Geometry: see drawing. Coordinates: mm, zero at the bounding-box minimum. A direction names the side the tool comes from. Give positions to 0.01 mm unless a question says otherwise; leave off trailing zeros. Loops run counter-clockwise (first coordinate to the right, second up) from the corner with the lowest first, then second, coordinate; pieces in that order, holes last. Notation, with made-up numbers: M 80,-32 L 87,-32 A23 cw 87,-12 Z; hole C 57.5,-39 d7. An arc over 180 degrees is marked long. Answer in a Markdown table with one row per item.
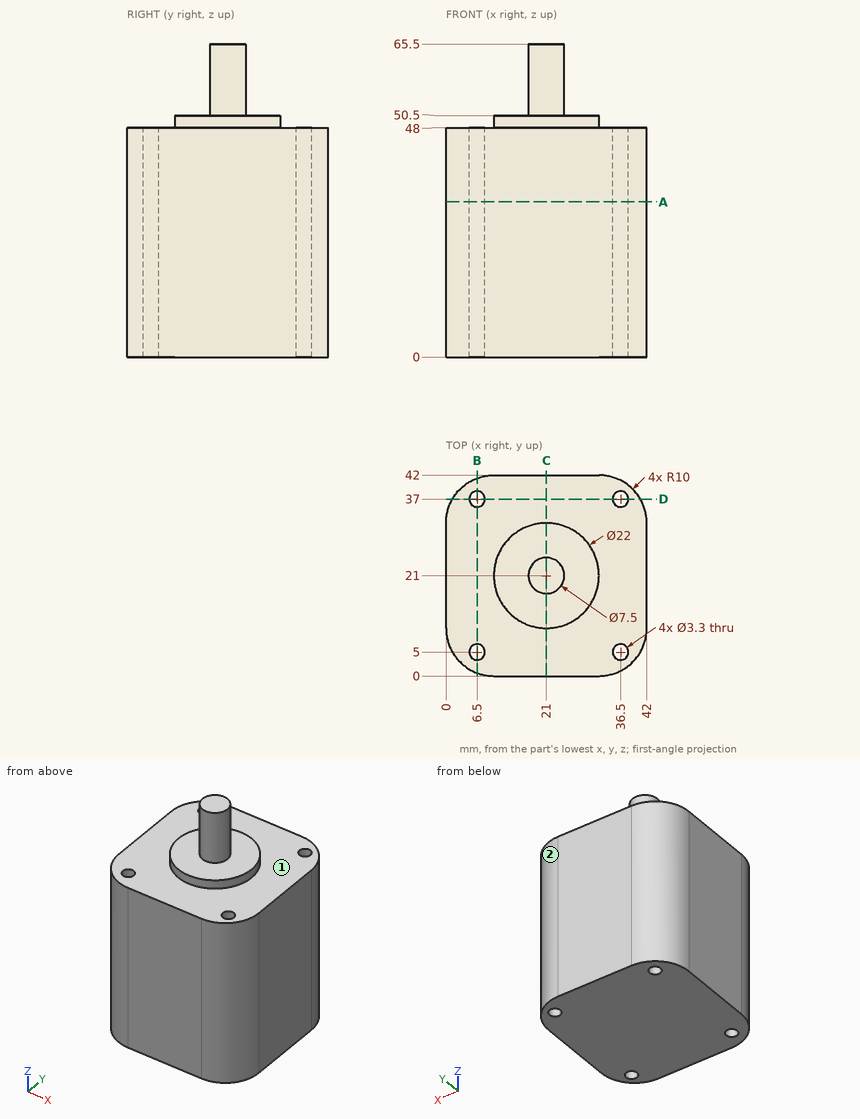
1) Material intervals for L1, parallel to Y at x = 36, z = 13; L2, parallel to X at y = 36.5, z = 17; L3, parallel to Y at x = 6.5, z = 34, sorted ascending.
Reply:
| item | result |
|---|---|
| L1 | y = 0.83 to 3.43, 6.57 to 35.43, 38.57 to 41.17 |
| L2 | x = 1.07 to 4.93, 8.07 to 34.93, 38.07 to 40.93 |
| L3 | y = 0.63 to 3.35, 6.65 to 35.35, 38.65 to 41.37 |
2) Section D-D, the plane y = 37. Return loops of the section in (x, z).
Reply:
| item | result |
|---|---|
| outline | M 1.34,0 L 4.85,0 L 4.85,48 L 1.34,48 Z; M 8.15,0 L 34.85,0 L 34.85,48 L 8.15,48 Z; M 38.15,0 L 40.66,0 L 40.66,48 L 38.15,48 Z |
3) Section B-B, the plane x = 6.5. Return loops of the section in (y, z), then the cut area to 3 significant figures.
Reply:
| item | result |
|---|---|
| outline | M 0.63,0 L 3.35,0 L 3.35,48 L 0.63,48 Z; M 6.65,0 L 35.35,0 L 35.35,48 L 6.65,48 Z; M 38.65,0 L 41.37,0 L 41.37,48 L 38.65,48 Z |
| area | 1,640 mm² |
4) Section A-A, the plane z = 32.5. Return loops of the section in (x, y).
Reply:
| item | result |
|---|---|
| outline | M 0,10 A10 ccw 10,0 L 32,0 A10 ccw 42,10 L 42,32 A10 ccw 32,42 L 10,42 A10 ccw 0,32 Z; hole C 6.5,5 d3.3; hole C 6.5,37 d3.3; hole C 36.5,5 d3.3; hole C 36.5,37 d3.3 |
5) Section C-C, the plane x = 21. Return loops of the section in (y, z), then the cut area to 3 significant figures.
Reply:
| item | result |
|---|---|
| outline | M 0,0 L 42,0 L 42,48 L 32,48 L 32,50.5 L 24.75,50.5 L 24.75,65.5 L 17.25,65.5 L 17.25,50.5 L 10,50.5 L 10,48 L 0,48 Z |
| area | 2,180 mm² |
6) Pin query (flat end, axial travel): pin 1 Ø2 at (x, z) = (6.5, 31) entering from -Y; pin 2 Ø2.5 at (x, y) = (6.5, 5) entering from -Z; pin 3 Ø8 at (x, y) = (4.5, 29.5) entering from +Z; pin 4 Ø12.5 at (x, y) = (30.5, 29) entering from +Z. Return the tip coordinate at first contact, or that it passes through.
Reply:
| item | result |
|---|---|
| pin 1 | stops at y = 0.32 |
| pin 2 | passes through |
| pin 3 | stops at z = 48 |
| pin 4 | stops at z = 50.5 |
7) Set-up query: the marked faces 1 and 2. Return all of +Z, -Z, +X, -X, +Y, -Y with unobstructed straight access to the full face (end or side cutting, diameter ignored); none if empty.
Reply:
| item | result |
|---|---|
| face 1 | +Z |
| face 2 | +Z, -Z, +X, +Y |
